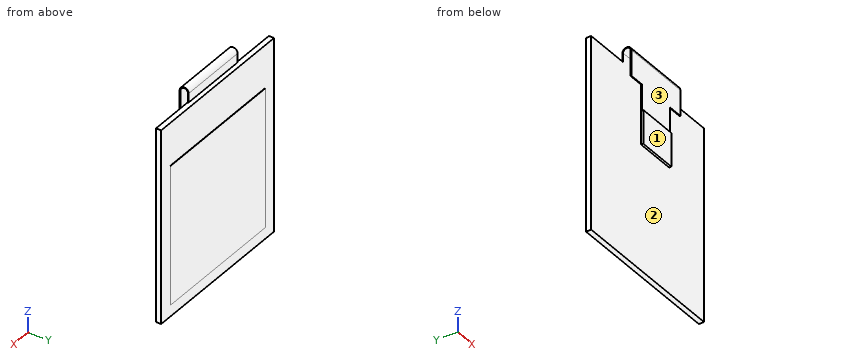
from build123d import *

# Parameters (mm, degrees)
SKETCH_1_W           = 22.12
SKETCH_1_H           = 25.82
SKETCH_1_W_2         = 18.56
SKETCH_1_H_2         = 18.56
EXTRUDE_1_DEPTH      = 0.7
SKETCH_1_2_W         = 18.56
SKETCH_1_2_H         = 18.56
EXTRUDE_2_DEPTH      = 0.745
EXTRUDE_3_DEPTH      = 4.8
EXTRUDE_3_DEPTH_BACK = 4.8
SKETCH_3_W           = 5.5
SKETCH_3_H           = 8
EXTRUDE_4_DEPTH      = 0.1
SKETCH_4_W           = 5.5
SKETCH_4_H           = 4.5
EXTRUDE_5_DEPTH      = 0.2


with BuildPart() as part:
    # 草图1 → 凸台-拉伸1 (new body)
    with BuildSketch(Plane(origin=(0, 0, 0), x_dir=(1, 0, 0), z_dir=(0, 1, 0))):
        with Locations((0, -2.08)):
            Rectangle(SKETCH_1_W, SKETCH_1_H)
        Rectangle(SKETCH_1_W_2, SKETCH_1_H_2, mode=Mode.SUBTRACT)
    extrude(amount=EXTRUDE_1_DEPTH)

    # 草图1<2> → 凸台-拉伸2 (add)
    with BuildSketch(Plane(origin=(0, 0, 0), x_dir=(1, 0, 0), z_dir=(0, 1, 0))):
        Rectangle(SKETCH_1_2_W, SKETCH_1_2_H)
    extrude(amount=EXTRUDE_2_DEPTH)

    # 草图2 → 凸台-拉伸3 (add, two sides: drawn at the far end of the back side and taken through both)
    with BuildSketch(Plane(origin=(0, 0, 0), x_dir=(0, 0, -1), z_dir=(1, 0, 0)).offset(-EXTRUDE_3_DEPTH_BACK)):
        with BuildLine():
            Line((-14.99, 0), (-16.19, 0))
            ThreePointArc((-16.19, 0), (-16.69, -0.5), (-16.19, -1))
            Line((-16.19, -1), (-12.76, -1))
            Line((-12.76, -1), (-12.76, -1.1))
            Line((-12.76, -1.1), (-16.19, -1.1))
            ThreePointArc((-16.19, -1.1), (-16.79, -0.5), (-16.19, 0.1))
            Line((-16.19, 0.1), (-14.99, 0.1))
            Line((-14.99, 0.1), (-14.99, 0))
        make_face()
    extrude(amount=EXTRUDE_3_DEPTH + EXTRUDE_3_DEPTH_BACK)

    # 草图3 → 凸台-拉伸4 (add)
    with BuildSketch(Plane.XZ.offset(1.1)):
        with Locations((0, 8.76)):
            Rectangle(SKETCH_3_W, SKETCH_3_H)
    extrude(amount=-EXTRUDE_4_DEPTH)

    # 草图4 → 凸台-拉伸5 (add)
    with BuildSketch(Plane.XZ.offset(1.1)):
        with Locations((0, 7.01)):
            Rectangle(SKETCH_4_W, SKETCH_4_H)
    extrude(amount=EXTRUDE_5_DEPTH)


solid = part.part
Geometry check sheet. Reference: the model listing, model coordinates, mm. Face numbers are marked on the shaded views. A direction names the side the tool comes from. Give positions to 0.01 mm unless a question says otherwise; leave off trailing zeros. Order: outer loops, then holes, each group sorted by start corner. A loop starts at its lowest first (then second) coordinate and runs counter-clockwise, first axis right, second up. Notation, with made-up numbers: M 78.5,35.5 L 84.5,35.5 A17 cw 84.5,52.5 Z; hole C 51,62 d2. An arc over 180 degrees is marked long. Use a Markdown table: item, result.
Item 1: Tool access check on the marked faces 1, 2 and 3. Record the directions out of +Z, -Z, +X, -X, +Y, -Y that give a thin tool (end or side, any length) a straight path to the whole face; none if there is none.
Answers follow:
| item | result |
|---|---|
| face 1 | +Z, -Z, +X, -X, -Y |
| face 2 | -Z, +X, -X |
| face 3 | +Z, +X, -X, -Y |
Item 2: Material ranges on line 1 along Z through (x, y) = (7.75, 0.35); line 2 along Y through (x, z) = (9, 6.25) (3 decimals); line 3 along Z through (x, y) = (2.5, -1.2), recorded low to high.
Answers follow:
| item | result |
|---|---|
| line 1 | z = -10.83 to 14.99 |
| line 2 | y = 0 to 0.745 |
| line 3 | z = 4.76 to 9.26 |
Item 3: Section check C-C (x = 1.5). Record the cut outline in (y, z) (3 decimals), and give its area (3 significant figures).
Answers follow:
| item | result |
|---|---|
| outline | M -1.3,4.76 L -1,4.76 L -1,16.19 A0.5 cw 0,16.19 L 0,-10.83 L 0.7,-10.83 L 0.7,-9.28 L 0.745,-9.28 L 0.745,9.28 L 0.7,9.28 L 0.7,14.99 L 0.1,14.99 L 0.1,16.19 A0.6 ccw -1.1,16.19 L -1.1,9.26 L -1.3,9.26 Z |
| area | 21.2 mm2 |
Item 4: Section check B-B (z = 5.75). Record the cut outline in (x, y) (3 decimals).
Answers follow:
| item | result |
|---|---|
| outline | M -11.06,0 L 11.06,0 L 11.06,0.7 L 9.28,0.7 L 9.28,0.745 L -9.28,0.745 L -9.28,0.7 L -11.06,0.7 Z; M -2.75,-1.3 L 2.75,-1.3 L 2.75,-1 L -2.75,-1 Z |
Item 5: Section check D-D (y = -0.5). Record the cut outline in (x, z).
Answers follow:
| item | result |
|---|---|
| outline | M -4.8,16.69 L 4.8,16.69 L 4.8,16.79 L -4.8,16.79 Z |
Item 6: Section check A-A (z = 10). Record the cut outline in (x, y), and give its area (3 significant figures).
Answers follow:
| item | result |
|---|---|
| outline | M -11.06,0 L 11.06,0 L 11.06,0.7 L -11.06,0.7 Z; M -2.75,-1.1 L 2.75,-1.1 L 2.75,-1 L -2.75,-1 Z |
| area | 16.0 mm2 |
Item 7: Depth check by flat-ended pin: P1, Ø2, axis at x = 0, z = 13.5, coming from the -Y side; P2, Ø1.3, axis at x = 0.5, z = 15.5, coming from the +Y side; P3, Ø3, axis at x = 7, z = 1.5, coming from the -Y side. Enter the tip coordinate at first touch or a pass-through.
Answers follow:
| item | result |
|---|---|
| P1 | stops at y = -1.1 |
| P2 | stops at y = 0.7 |
| P3 | stops at y = 0 |
